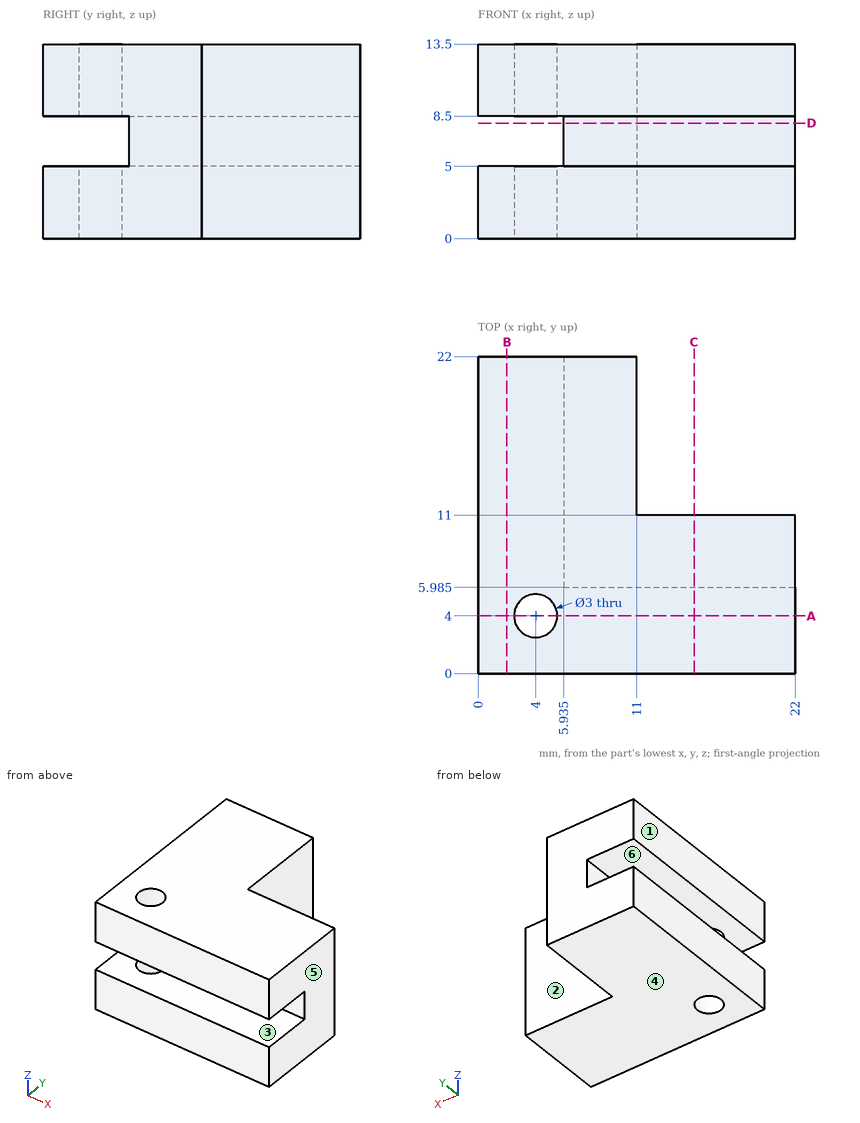
Design review of the part shown in the three views and the two pictorial views. Dimensions are in mm from the part's minimum x, y and z. A direction names the side the tool comes from. Give positions to 0.01 mm unless a question says otherwise; leave off trailing zeros. Loops run counter-clockwise (first coordinate to the right, second up) from the corner with the lowest first, then second, coordinate; pieces in that order, holes last. Notation, with made-up numbers: (66.25, 3.5) -> (103.25, 3.5) arc R26 ccw to (103.25, 25.5) -> close; hole circle Ø4 at (79, 20). An arc over 180 degrees is marked (long way). Put each result on its own line as item: value. Start each with the question number.
1. Clearance check with flat-ended pins moving along their axes: P1, Ø8, axis at x = 16.5, y = 18.5, coming from the +Z side; P2, Ø3.5, axis at x = 15.5, z = 5, coming from the +Y side. State where each tip first meets the part, or that it passes through.
2. We need section B-B on x = 2. State the section outline as (y, z) points.
3. For the marked faces 1 and 2, list the 3-axis set-ups (+Z, -Z, +X, -X, +Y, -Y) from which the entire face can be reached by the end or side of a thin tool; tool diameter is ignored.
4. We need section C-C on x = 15. State the section outline as (y, z) points (1 decimal).
5. Wall thickness on probe 1 along Y at (x, z) = (4, 11.8); probe 2 along Z at (x, y) = (1, 7.75): over which ranges is each line inside the solid? List them lowest first.
6. We need section A-A on y = 4. State the section outline as (x, z) points, then the cut area to 3 significant figures.
7. We need section D-D on z = 8. State the section outline as (x, y) points (1 decimal).
8. Mouldability with a two-part tool opening along Z and no side actions: class the marked faces 3, 4, 5 and 6 as released by +Z, released by -Z, zero draft, split by the parting line, or undercut.
Determined:
1. P1: through
1. P2: y = 11
2. outline: (0, 0) -> (22, 0) -> (22, 5) -> (0, 5) -> close; (0, 8.5) -> (22, 8.5) -> (22, 13.5) -> (0, 13.5) -> close
3. face 1: +Z, -Z, -X, +Y, -Y
3. face 2: +Z, -Z, +X, +Y
4. outline: (0, 0) -> (11, 0) -> (11, 13.5) -> (0, 13.5) -> (0, 8.5) -> (6, 8.5) -> (6, 5) -> (0, 5) -> close
5. probe 1: 0 to 2.5, 5.5 to 22
5. probe 2: 0 to 5, 8.5 to 13.5
6. outline: (0, 0) -> (2.5, 0) -> (2.5, 5) -> (0, 5) -> close; (0, 8.5) -> (2.5, 8.5) -> (2.5, 13.5) -> (0, 13.5) -> close; (5.5, 0) -> (22, 0) -> (22, 5) -> (5.5, 5) -> close; (5.5, 8.5) -> (22, 8.5) -> (22, 13.5) -> (5.5, 13.5) -> close
6. area: 190 mm^2
7. outline: (5.9, 6) -> (22, 6) -> (22, 11) -> (11, 11) -> (11, 22) -> (5.9, 22) -> close
8. face 3: undercut
8. face 4: released by -Z
8. face 5: zero draft
8. face 6: undercut
